Job drawing, mm, ordinate dimensions from the low corner. One solid piece. Coordinates: 2 decimals unless noted, no trailing zeros. Order: outer loops, then holes, each group sorted by start corner. A loop starts at its lowest first (then second) coordinate and runs counter-clockwise, first axis right, second up. Notation, with made-up numbers: M 35,47 L 45,47 A20 cw 45,53 Z; hole C 35.25,34.5 d2. An arc over 180 degrees is marked long. Write item = value, one per line. Start each with the question number.
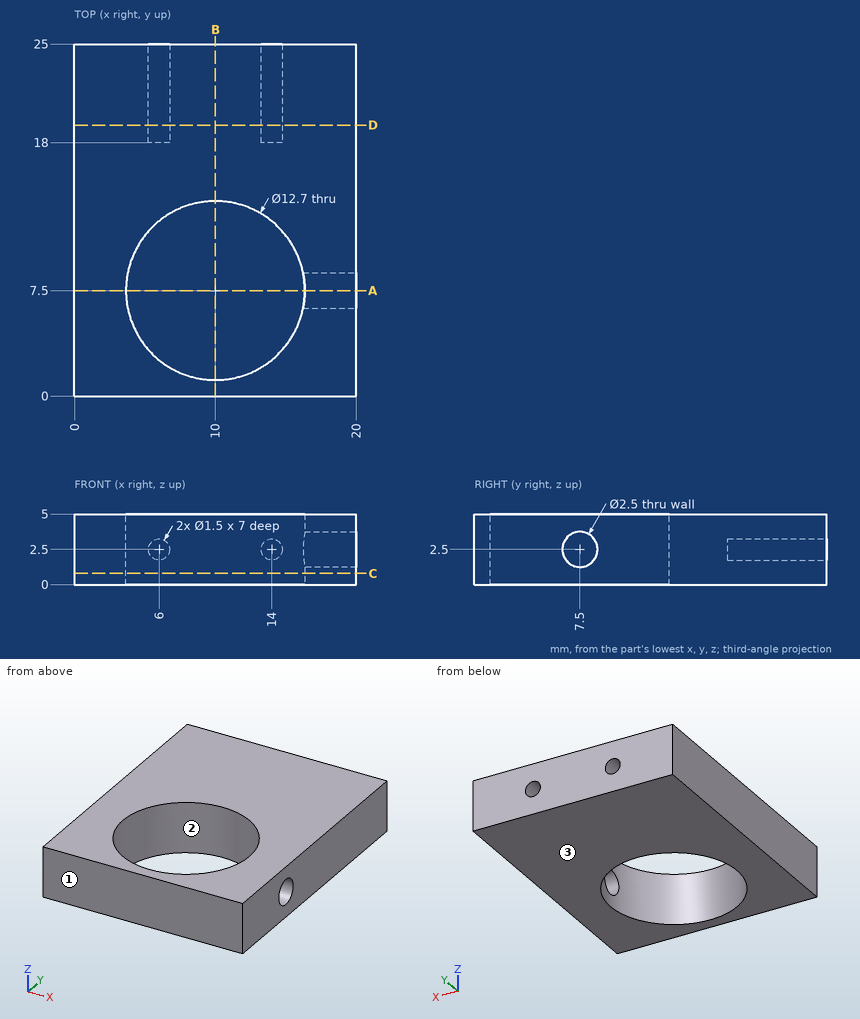
1. Flat gauge pin, fed straight in: pin 1 (1.2 mm diameter, centred on x = 14, z = 2.5, fed in from +Y). Where does the tip first touch, or does it go through?
2. Slice it at B-B (x = 10). Write the cut outline in (y, z).
3. Slice it at D-D (y = 19.25). Write the cut outline in (x, z), plus the area to 3 significant figures.
4. Probe L1, parallel to Z at x = 14, y = 22.25; L2, parallel to X at y = 7.25, z = 3.9; L3, parallel to Y at x = 10, z = 3.7. List the from-to ranges inside material, lowest first.
5. Slice it at C-C (z = 0.8). Write the cut outline in (x, y), plus the area to 3 significant figures.
6. Mould opens along Y. For the marked faces 1, 2 and 3 say: released by +Y, released by -Y, zero draft, split by the parting line, or undercut.
7. Slice it at A-A (y = 7.5). Write the cut outline in (x, z), plus the area to 3 significant figures.
Calculated:
q1.pin_1 = 18
q2.outline = M 0,0 L 1.15,0 L 1.15,5 L 0,5 Z; M 13.85,0 L 25,0 L 25,5 L 13.85,5 Z
q3.outline = M 0,0 L 20,0 L 20,5 L 0,5 Z; hole C 6,2.5 d1.5; hole C 14,2.5 d1.5
q3.area = 96.5 mm²
q4.L1 = 0 to 1.75, 3.25 to 5
q4.L2 = 0 to 3.65, 16.35 to 20
q4.L3 = 0 to 1.15, 13.85 to 25
q5.outline = M 0,0 L 20,0 L 20,25 L 0,25 Z; hole C 10,7.5 d12.7
q5.area = 373 mm²
q6.face_1 = released by -Y
q6.face_2 = undercut
q6.face_3 = zero draft
q7.outline = M 0,0 L 3.65,0 L 3.65,5 L 0,5 Z; M 16.35,0 L 20,0 L 20,1.25 L 16.35,1.25 Z; M 16.35,3.75 L 20,3.75 L 20,5 L 16.35,5 Z
q7.area = 27.4 mm²
